Geometry check sheet. Reference: the model listing, model coordinates, mm. Give positions to 0.01 mm unless a question says otherwise; leave off trailing zeros. Order: outer loops, then holes, each group sorted by start corner. A loop starts at its lowest first (then second) coordinate and runs counter-clockwise, first axis right, second up. Notation, with made-up numbers: (9, 4.25) - (50, 4.25) arc R19 cw to (50, 35.25) - close; hole circle Ø2 at (44.5, 1.5). An arc over 180 degrees is marked (long way). Put each result on its own line as item: value. Start each with the question number.
```python
from build123d import *

# Parameters (mm, degrees)
SKETCH1_R           = 41
BOSS_EXTRUDE1_DEPTH = 18.4
SKETCH2_R           = 39.5
BOSS_EXTRUDE2_DEPTH = 2
SKETCH3_R           = 41
BOSS_EXTRUDE3_DEPTH = 5
SKETCH4_R           = 2.5
CUT_EXTRUDE1_DEPTH  = 5
CUT_EXTRUDE2_START  = -3
SKETCH5_R           = 2.5
CUT_EXTRUDE2_DEPTH  = 3


with BuildPart() as part:
    # Sketch1 → Boss-Extrude1 (new body)
    with BuildSketch(Plane(origin=(0, 0, 0), x_dir=(1, 0, 0), z_dir=(0, 1, 0))):
        with Locations(Location((0, 0, 0), (0, 0, 270))):
            Circle(SKETCH1_R)
    extrude(amount=BOSS_EXTRUDE1_DEPTH)

    # Sketch2 → Boss-Extrude2 (add)
    with BuildSketch(Plane(origin=(0, 18.4, 0), x_dir=(1, 0, 0), z_dir=(0, 1, 0))):
        with Locations(Location((0, 0, 0), (0, 0, 270))):
            Circle(SKETCH2_R)
    extrude(amount=BOSS_EXTRUDE2_DEPTH)

    # Sketch3 → Boss-Extrude3 (add)
    with BuildSketch(Plane(origin=(0, 20.4, 0), x_dir=(1, 0, 0), z_dir=(0, 1, 0))):
        with Locations(Location((0, 0, 0), (0, 0, 270))):
            Circle(SKETCH3_R)
    extrude(amount=BOSS_EXTRUDE3_DEPTH)

    # Sketch4 → Cut-Extrude1 (cut)
    with BuildSketch(Plane.XZ):
        with Locations(Location((30.795863359, 17.78, 0), (0, 0, 270))):
            Circle(SKETCH4_R)
        with Locations(Location((30.795863359, -17.78, 0), (0, 0, 270))):
            Circle(SKETCH4_R)
        with Locations(Location((0, -35.56, 0), (0, 0, 270))):
            Circle(SKETCH4_R)
        with Locations(Location((-30.795863359, -17.78, 0), (0, 0, 270))):
            Circle(SKETCH4_R)
        with Locations(Location((-30.795863359, 17.78, 0), (0, 0, 270))):
            Circle(SKETCH4_R)
        with Locations(Location((0, 35.56, 0), (0, 0, 270))):
            Circle(SKETCH4_R)
    extrude(amount=-CUT_EXTRUDE1_DEPTH, mode=Mode.SUBTRACT)

    # Sketch5 → Cut-Extrude2 (cut)
    with BuildSketch(Plane(origin=(0, 25.4, 0), x_dir=(1, 0, 0), z_dir=(0, 1, 0)).offset(CUT_EXTRUDE2_START)):
        with Locations(Location((30.795863359, 17.78, 0), (0, 0, 90))):
            Circle(SKETCH5_R)
        with Locations(Location((30.795863359, -17.78, 0), (0, 0, 90))):
            Circle(SKETCH5_R)
        with Locations(Location((0, -35.56, 0), (0, 0, 90))):
            Circle(SKETCH5_R)
        with Locations(Location((-30.795863359, -17.78, 0), (0, 0, 90))):
            Circle(SKETCH5_R)
        with Locations(Location((-30.795863359, 17.78, 0), (0, 0, 90))):
            Circle(SKETCH5_R)
        with Locations(Location((0, 35.56, 0), (0, 0, 90))):
            Circle(SKETCH5_R)
    extrude(amount=CUT_EXTRUDE2_DEPTH, mode=Mode.SUBTRACT)


solid = part.part
```
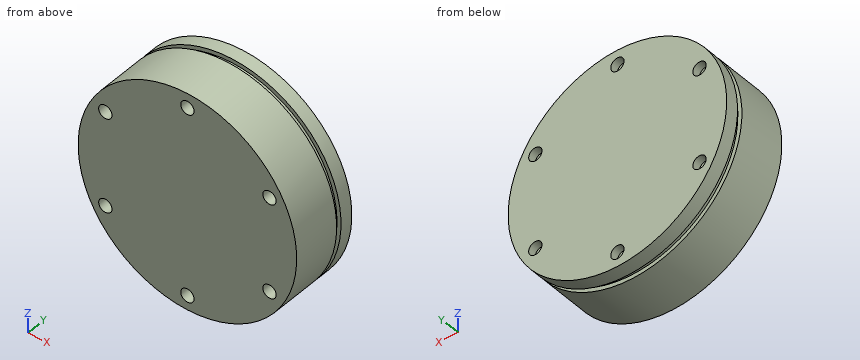
Item 1: Gauge pin test, flat ends, axial feed: pin 1 Ø6 at (x, y) = (30, 6.5) entering from -Z; pin 2 Ø3 at (y, z) = (14.5, -27.5) entering from +X; pin 3 Ø1.5 at (x, y) = (-5, 13.5) entering from +Z. Record the tip position at first contact, or that the pin passes through.
Item 2: Cross-section at D-D (y = 16). Enter the section's corners in (x, z), and give its area (3 significant figures).
Item 3: Thickness scan on line 1 along X through (y, z) = (24.5, -17.78); line 2 along X through (y, z) = (2, -35.56); line 3 along X through (y, z) = (19.25, 0.5). Record the ranges inside material, lowest first.
Item 4: Cross-section at B-B (z = 30). Enter the section's corners in (x, y).
Item 5: Cross-section at C-C (y = 2.5). Enter the section's corners in (x, z).
Item 6: Cross-section at A-A (x = 0). Enter the section's corners in (y, z), and give its area (3 significant figures).
Recorded:
1. pin 1: stops at z = -30.85
1. pin 2: stops at x = 31.7
1. pin 3: stops at z = 40.78
2. outline: circle Ø82 at (0, 0)
2. area: 5,280 mm^2
3. line 1: x = -36.94 to -33.3, -28.3 to 28.3, 33.3 to 36.94
3. line 2: x = -20.41 to -2.5, 2.5 to 20.41
3. line 3: x = -39.5 to 39.5
4. outline: (-27.95, 0) - (27.95, 0) - (27.95, 18.4) - (25.7, 18.4) - (25.7, 20.4) - (27.95, 20.4) - (27.95, 25.4) - (-27.95, 25.4) - (-27.95, 20.4) - (-25.7, 20.4) - (-25.7, 18.4) - (-27.95, 18.4) - close
5. outline: circle Ø82 at (0, 0); hole circle Ø5 at (-30.8, -17.78); hole circle Ø5 at (-30.8, 17.78); hole circle Ø5 at (0, -35.56); hole circle Ø5 at (0, 35.56); hole circle Ø5 at (30.8, -17.78); hole circle Ø5 at (30.8, 17.78)
6. outline: (0, -41) - (18.4, -41) - (18.4, -39.5) - (20.4, -39.5) - (20.4, -41) - (25.4, -41) - (25.4, -38.06) - (22.4, -38.06) - (22.4, -33.06) - (25.4, -33.06) - (25.4, 33.06) - (22.4, 33.06) - (22.4, 38.06) - (25.4, 38.06) - (25.4, 41) - (20.4, 41) - (20.4, 39.5) - (18.4, 39.5) - (18.4, 41) - (0, 41) - (0, 38.06) - (5, 38.06) - (5, 33.06) - (0, 33.06) - (0, -33.06) - (5, -33.06) - (5, -38.06) - (0, -38.06) - close
6. area: 2,000 mm^2
